```python
from build123d import *

# Parameters (mm, degrees)
F0_W     = 101.6
F0_H     = 101.6
F1_DEPTH = 6.35
F2_W     = 6.35
F2_H     = 88.9
F3_DEPTH = 38.1
F4_W     = 44.45
F4_H     = 44.45
F4_R     = 19.685
F5_DEPTH = 30.48


with BuildPart() as f1:
    # F0 (on Top) → F1 (new body)
    with BuildSketch(Plane.XY):
        Rectangle(F0_W, F0_H)
    extrude(amount=F1_DEPTH)

    # F2 (on face) → F3 (join)
    with BuildSketch(Plane.XY.offset(6.35)):
        Polygon((50.8, 50.8), (-50.8, 50.8), (-50.8, 44.45), (-44.45, 44.45), (44.45, 44.45), (50.8, 44.45), align=None)
        with Locations((-47.625, 0)):
            Rectangle(F2_W, F2_H)
        Polygon((50.8, -50.8), (50.8, 44.45), (44.45, 44.45), (44.45, -44.45), (44.45, -50.8), align=None)
        Polygon((-44.45, -44.45), (-50.8, -44.45), (-50.8, -50.8), (44.45, -50.8), (44.45, -44.45), align=None)
    extrude(amount=F3_DEPTH)

    # F4 (on face) → F5 (join)
    with BuildSketch(Plane.XY.offset(6.35)):
        with Locations((-22.225, 22.225)):
            Rectangle(F4_W, F4_H)
        with Locations((-22.225, 22.225)):
            Circle(F4_R, mode=Mode.SUBTRACT)
        with Locations((22.225, 22.225)):
            Rectangle(F4_W, F4_H)
        with Locations((22.225, 22.225)):
            Circle(F4_R, mode=Mode.SUBTRACT)
        with Locations((22.225, -22.225)):
            Rectangle(F4_W, F4_H)
        with Locations((22.225, -22.225)):
            Circle(F4_R, mode=Mode.SUBTRACT)
        with Locations((-22.225, -22.225)):
            Rectangle(F4_W, F4_H)
        with Locations((-22.225, -22.225)):
            Circle(F4_R, mode=Mode.SUBTRACT)
    extrude(amount=F5_DEPTH)


solid = f1.part
```
Source: CAD feature listing. Evaluate the final solid. Frame: model axes, mm. A direction names the side the tool comes from. Give positions to 0.01 mm unless a question says otherwise; leave off trailing zeros. Loops run counter-clockwise (first coordinate to the right, second up) from the corner with the lowest first, then second, coordinate; pieces in that order, holes last. Notation, with made-up numbers: (30, -39) -> (78, -39) arc R23 cw to (78, -1) -> close; hole circle Ø6 at (63.5, 33.5). An arc over 180 degrees is marked (long way). Use a Markdown table: item, result. Add a question column.
(1) Ray query, line 1 (Y direction, x = -12, z = 40); line 2 (X direction, y = -34.5, z = 24.5); line 3 (Y direction, x = -19.5, z = 24). Return the intervals inside material, ascending.
(2) Access query for faces 1 (the face through (-50.8, 1, 22)), 2 (the face through (-3.45, -16.31, 21.38)). Directions: +Z, -Z, +X, -X, +Y, -Y. A direction counts if a zero-diameter tool reaches every point of the face in a straight line with its end or side. Return the directions, or none.
(3) Section query B-B (z = 8). Output: boundary loops of the cut face in (x, y) (3 decimals).
(4) Section query D-D (y = -19). Output: boundary loops of the cut face in (x, z), then the cut area to 3 significant figures.
(5) Section query A-A (y = -1). Output: boundary loops of the cut face in (x, z), then the cut area to 3 significant figures.
(6) First-contact query: pin 1 Ø12 at (x, y) = (19.5, -20) entering from +Z; pin 2 Ø23.5 at (x, y) = (22.225, -22.225) entering from -Z. Flat tips, straight axial feed; report the tip coordinate or a pass-through.
(7) Section query C-C (x = -6.5). Output: boundary loops of the cut face in (y, z).
(8) Pull-direction query (Y, two-part tool) for faces 3 (the face through (-23, -22, 6.35)), 4 (the face through (-1, 1, 0)), 5 (the face through (-1, -50.8, 22)); classes: +Y half, -Y half, draft (parallel to the pull), parting line (faces both ways), or undercut.
Checked values:
| question | item | result |
|---|---|---|
| 1 | line 1 | -50.8 to -44.45, 44.45 to 50.8 |
| 1 | line 2 | -50.8 to -37.61, -6.84 to 6.84, 37.61 to 50.8 |
| 1 | line 3 | -50.8 to -41.72, -2.73 to 2.73, 41.72 to 50.8 |
| 2 | face 1 | +Z, -Z, -X, +Y, -Y |
| 2 | face 2 | +Z |
| 3 | outline | (-50.8, -50.8) -> (50.8, -50.8) -> (50.8, 50.8) -> (-50.8, 50.8) -> close; hole circle Ø39.37 at (-22.225, -22.225); hole circle Ø39.37 at (-22.225, 22.225); hole circle Ø39.37 at (22.225, -22.225); hole circle Ø39.37 at (22.225, 22.225) |
| 4 | outline | (-50.8, 0) -> (50.8, 0) -> (50.8, 44.45) -> (44.45, 44.45) -> (44.45, 36.83) -> (41.64, 36.83) -> (41.64, 6.35) -> (2.81, 6.35) -> (2.81, 36.83) -> (-2.81, 36.83) -> (-2.81, 6.35) -> (-41.64, 6.35) -> (-41.64, 36.83) -> (-44.45, 36.83) -> (-44.45, 44.45) -> (-50.8, 44.45) -> close |
| 4 | area | 1,470 mm^2 |
| 5 | outline | (-50.8, 0) -> (50.8, 0) -> (50.8, 44.45) -> (44.45, 44.45) -> (44.45, 36.83) -> (-44.45, 36.83) -> (-44.45, 44.45) -> (-50.8, 44.45) -> close |
| 5 | area | 3,840 mm^2 |
| 6 | pin 1 | z = 6.35 |
| 6 | pin 2 | z = 0 |
| 7 | outline | (-50.8, 0) -> (50.8, 0) -> (50.8, 44.45) -> (44.45, 44.45) -> (44.45, 36.83) -> (34.07, 36.83) -> (34.07, 6.35) -> (10.38, 6.35) -> (10.38, 36.83) -> (-10.38, 36.83) -> (-10.38, 6.35) -> (-34.07, 6.35) -> (-34.07, 36.83) -> (-44.45, 36.83) -> (-44.45, 44.45) -> (-50.8, 44.45) -> close |
| 8 | face 3 | undercut |
| 8 | face 4 | draft |
| 8 | face 5 | -Y half |
